from build123d import *
from OCP.BRepFilletAPI import BRepFilletAPI_MakeChamfer

# Parameters (mm, degrees)
BOSS_EXTRU_1_DEPTH           = 3
BOSS_EXTRU_2_DEPTH           = 3
ENL_V_MAT_EXTRU_1_DEPTH      = 69.745908969
ENL_V_MAT_EXTRU_1_DEPTH_BACK = 69.745908969
ESQUISSE3_W                  = 34
ESQUISSE3_H                  = 7
ESQUISSE4_R                  = 1.75
ENL_V_MAT_EXTRU_2_DEPTH      = 2
ESQUISSE5_R                  = 1
ENL_V_MAT_EXTRU_3_DEPTH      = 1
ESQUISSE6_W                  = 1.5
ESQUISSE6_H                  = 3
ESQUISSE6_W_2                = 3
ESQUISSE6_H_2                = 1.5
BOSS_EXTRU_3_DEPTH           = 1.5
CHANFREIN1_SIZE              = 1.4
CHANFREIN1_SIZE2             = 2.633017051
SYM_TRIE1_START              = 3.5
SYM_TRIE1_DEPTH              = 1.5


# Read off the part's stored shape, not the designer's step: Symétrie1
with BuildPart() as part:
    # Esquisse1 → Boss.-Extru.1 (new body)
    with BuildSketch(Plane.XY):
        Polygon((0, 0), (5, -5), (46, -5), (51, 0), (51, 41), (46, 46), (5, 46), (0, 41), align=None)
    extrude(amount=BOSS_EXTRU_1_DEPTH)

    # Esquisse2 → Boss.-Extru.2 (add)
    with BuildSketch(Plane.XY.offset(3)):
        Polygon((5, 41), (5, 34), (3.5, 32.5), (3.5, 42.5), (13.5, 42.5), (12, 41), align=None)
        Polygon((3.5, -1.5), (13.5, -1.5), (12, 0), (5, 0), (5, 7), (3.5, 8.5), align=None)
        Polygon((47.5, 42.5), (47.5, 32.5), (46, 34), (46, 41), (39, 41), (37.5, 42.5), align=None)
        Polygon((46, 7), (46, 0), (39, 0), (37.5, -1.5), (47.5, -1.5), (47.5, 8.5), align=None)
    extrude(amount=BOSS_EXTRU_2_DEPTH)

    # Esquisse3 → Enlèv. mat.-Extru.1 (cut, two sides: drawn at the far end of the back side and taken through both)
    with BuildSketch(Plane.XY.offset(3).offset(-ENL_V_MAT_EXTRU_1_DEPTH_BACK)):
        with Locations((25.5, -1.5)):
            Rectangle(ESQUISSE3_W, ESQUISSE3_H)
    extrude(amount=ENL_V_MAT_EXTRU_1_DEPTH + ENL_V_MAT_EXTRU_1_DEPTH_BACK, mode=Mode.SUBTRACT)

    # Esquisse4 → Enlèv. mat.-Extru.2 (cut)
    with BuildSketch(Plane(origin=(0, 0, 0), x_dir=(-1, 0, 0), z_dir=(0, 0, -1))):
        with Locations((-25.5, 43.75)):
            Circle(ESQUISSE4_R)
        with Locations((-48.75, 20.5)):
            Circle(ESQUISSE4_R)
        with Locations((-2.25, 20.5)):
            Circle(ESQUISSE4_R)
    extrude(amount=-ENL_V_MAT_EXTRU_2_DEPTH, mode=Mode.SUBTRACT)

    # Esquisse5 → Enlèv. mat.-Extru.3 (cut)
    with BuildSketch(Plane(origin=(0, 0, 2), x_dir=(-1, 0, 0), z_dir=(0, 0, -1))):
        with Locations((-25.5, 43.75)):
            Circle(ESQUISSE5_R)
        with Locations((-2.25, 20.5)):
            Circle(ESQUISSE5_R)
        with Locations((-48.75, 20.5)):
            Circle(ESQUISSE5_R)
    extrude(amount=-ENL_V_MAT_EXTRU_3_DEPTH, mode=Mode.SUBTRACT)

    # Esquisse6 → Boss.-Extru.3 (add)
    with BuildSketch(Plane.XY.offset(6)):
        with Locations((9.25, 41)):
            Rectangle(ESQUISSE6_W, ESQUISSE6_H)
        with Locations((41.75, 41)):
            Rectangle(ESQUISSE6_W, ESQUISSE6_H)
        with Locations((5, 36.75)):
            Rectangle(ESQUISSE6_W_2, ESQUISSE6_H_2)
        with Locations((46, 36.75)):
            Rectangle(ESQUISSE6_W_2, ESQUISSE6_H_2)
    extrude(amount=BOSS_EXTRU_3_DEPTH)

    # Chanfrein1: one chamfer whose edges measure the first distance from different faces: ONE call of the kernel's chamfer builder (chamfer() names one face for all edges)
    chanfrein1_edges_1 = [part.edges().sort_by_distance(p)[0] for p in [
        (9.25, 39.5, 7.5),
    ]]
    chanfrein1_side_1 = [part.faces().sort_by_distance(p)[0] for p in [
        (9.25, 39.5, 6.75),
    ]]
    chanfrein1_edges_2 = [part.edges().sort_by_distance(p)[0] for p in [
        (41.75, 39.5, 7.5),
    ]]
    chanfrein1_side_2 = [part.faces().sort_by_distance(p)[0] for p in [
        (41.75, 39.5, 6.75),
    ]]
    chanfrein1_edges_3 = [part.edges().sort_by_distance(p)[0] for p in [
        (6.5, 36.75, 7.5),
    ]]
    chanfrein1_side_3 = [part.faces().sort_by_distance(p)[0] for p in [
        (6.5, 36.75, 6.75),
    ]]
    chanfrein1_edges_4 = [part.edges().sort_by_distance(p)[0] for p in [
        (44.5, 36.75, 7.5),
    ]]
    chanfrein1_side_4 = [part.faces().sort_by_distance(p)[0] for p in [
        (44.5, 36.75, 6.75),
    ]]
    chanfrein1 = BRepFilletAPI_MakeChamfer(part.part.solid().wrapped)
    for e in chanfrein1_edges_1:
        chanfrein1.Add(CHANFREIN1_SIZE, CHANFREIN1_SIZE2, e.wrapped, chanfrein1_side_1[0].wrapped)  # the first distance lies on this face
    for e in chanfrein1_edges_2:
        chanfrein1.Add(CHANFREIN1_SIZE, CHANFREIN1_SIZE2, e.wrapped, chanfrein1_side_2[0].wrapped)  # the first distance lies on this face
    for e in chanfrein1_edges_3:
        chanfrein1.Add(CHANFREIN1_SIZE, CHANFREIN1_SIZE2, e.wrapped, chanfrein1_side_3[0].wrapped)  # the first distance lies on this face
    for e in chanfrein1_edges_4:
        chanfrein1.Add(CHANFREIN1_SIZE, CHANFREIN1_SIZE2, e.wrapped, chanfrein1_side_4[0].wrapped)  # the first distance lies on this face
    add(Compound.cast(chanfrein1.Shape()), mode=Mode.REPLACE)

    # Symétrie1 outline → Symétrie1 (add)
    with BuildSketch(Plane(origin=(0, 0, 0), x_dir=(1, 0, 0), z_dir=(0, 1, 0)).offset(SYM_TRIE1_START)):
        Polygon((3.5, -6), (3.5, -7.5), (3.866982949, -7.5), (6.5, -6.1), (6.5, -6), align=None)
        Polygon((47.5, -6), (44.5, -6), (44.5, -6.1), (47.133017051, -7.5), (47.5, -7.5), align=None)
    extrude(amount=SYM_TRIE1_DEPTH)


solid = part.part
Input: part model. Units: mm. Frame: model coordinates. A direction names the side the tool comes from. Give positions to 0.01 mm unless a question says otherwise; leave off trailing zeros. Order: outer loops, then holes, each group sorted by start corner. A loop starts at its lowest first (then second) coordinate and runs counter-clockwise, first axis right, second up.
Q1. Section B-B on z = 4.75. Output: boundary loops of the cut face in (x, y).
Checked values:
outline: (3.5, -1.5) - (8.5, -1.5) - (8.5, 0) - (5, 0) - (5, 7) - (3.5, 8.5) - close; (3.5, 32.5) - (5, 34) - (5, 41) - (12, 41) - (13.5, 42.5) - (3.5, 42.5) - close; (37.5, 42.5) - (39, 41) - (46, 41) - (46, 34) - (47.5, 32.5) - (47.5, 42.5) - close; (42.5, -1.5) - (47.5, -1.5) - (47.5, 8.5) - (46, 7) - (46, 0) - (42.5, 0) - close
Q2. Section A-A on y = 43.75. Output: boundary loops of the cut face in (x, z), and give its area (4 significant figures).
Checked values:
outline: (2.75, 0) - (23.75, 0) - (23.75, 2) - (24.5, 2) - (24.5, 3) - (2.75, 3) - close; (26.5, 2) - (27.25, 2) - (27.25, 0) - (48.25, 0) - (48.25, 3) - (26.5, 3) - close
area: 127.5 mm2
Q3. Section D-D on y = 20.5. Output: boundary loops of the cut face in (x, z), and give its area (3 significant figures).
Checked values:
outline: (0, 0) - (0.5, 0) - (0.5, 2) - (1.25, 2) - (1.25, 3) - (0, 3) - close; (3.25, 2) - (4, 2) - (4, 0) - (47, 0) - (47, 2) - (47.75, 2) - (47.75, 3) - (3.25, 3) - close; (49.75, 2) - (50.5, 2) - (50.5, 0) - (51, 0) - (51, 3) - (49.75, 3) - close
area: 135 mm2
Q4. Set-up query: faces 1 (the flat face through (1, 20, 2)), 2 (the flat face through (7, 0, 4)), 3 (the flat face through (47, 35, 6)). Return all of +Z, -Z, +X, -X, +Y, -Y with unobstructed straight access to the full face (end or side cutting, diameter ignored); none if empty.
Checked values:
face 1: -Z
face 2: +Z
face 3: +Z, +X, -X
Q5. Section C-C on x = 25.5. Output: boundary loops of the cut face in (y, z), and give its area (3 significant figures).
Checked values:
outline: (2, 0) - (42, 0) - (42, 2) - (42.75, 2) - (42.75, 3) - (2, 3) - close; (44.75, 2) - (45.5, 2) - (45.5, 0) - (46, 0) - (46, 3) - (44.75, 3) - close
area: 123 mm2
Q6. Draft query along Y for faces 4 (the flat face through (11, 42, 6)), 5 (the flat face through (46.3, 5, 6.6)), 6 (the cylindrical face through (47.809, 21.976, 0.986)), 7 (the flat face through (25, 2, 1)). Return one class per face: +Y half, -Y half, draft (parallel to the pull), parting line (faces both ways), or undercut.
Checked values:
face 4: draft
face 5: undercut
face 6: undercut
face 7: -Y half
Q7. Ray query, probe 1 along Y at (x, z) = (25.5, 0.4); probe 2 along Z at (x, y) = (3, 32.5); probe 3 along Y at (x, z) = (32, 2.5). Return the intervals inside material, ascending.
Checked values:
probe 1: y = 2 to 42, 45.5 to 46
probe 2: z = 0 to 3
probe 3: y = 2 to 46
Q8. Contact query for flat-ended pins moving along their axis: pin 1 Ø0.9 at (x, z) = (41, 4.5) entering from -Y; pin 2 Ø0.8 at (x, y) = (38.5, 41.5) entering from +Z; pin 3 Ø10 at (x, y) = (9.5, 8.5) entering from +Z. Output: stop coordinate, or through.
Checked values:
pin 1: stops at y = 41
pin 2: stops at z = 6
pin 3: stops at z = 6.4
